from build123d import *

# Parameters (mm, degrees)
FILLET1_R = 0.635


with BuildPart() as part:
    # Sketch1 → Body (revolve)
    with BuildSketch(Plane.XY, mode=Mode.PRIVATE) as body_sk:
        with BuildLine():
            Line((-0.2794, 5.0038), (0, 5.0038))
            Line((0, 5.0038), (0, 2.38125))
            Line((0, 2.38125), (9.526, 2.38125))
            Line((9.526, 2.38125), (9.526, 3.602736))
            ThreePointArc((9.526, 3.602736), (11.862096638, 3.446669338), (14.098, 2.75209))
            Line((14.098, 2.75209), (14.098, 0))
            Line((14.098, 0), (-1.524, 0))
            ThreePointArc((-1.524, 0), (-1.208180863, 2.578131281), (-0.2794, 5.0038))
        make_face()
    revolve(body_sk.sketch.rotate(Axis((-1.524, 0, 0), (1, 0, 0)), 180), axis=Axis((-1.524, 0, 0), (1, 0, 0)))

    # Fillet1
    fillet1_edges = [part.edges().sort_by_distance(p)[0] for p in [
        (0, 2.38125, 0),
    ]]
    fillet(fillet1_edges, radius=FILLET1_R)


solid = part.part
Read the model definition and answer for the solid it produces. Units are mm, in the model's axes. Give positions to 0.01 mm unless a question says otherwise; leave off trailing zeros. Write each loop counter-clockwise with the first axis right and the second up, starting at its lowest first coordinate (ties: lowest second). Pieces come first, ordered by that corner, then holes. Notation, with made-up numbers: (69, 60) - (86, 60) arc R27 ccw to (86, 80) - close; hole circle Ø2 at (-33, -7.75). An arc over 180 degrees is marked (long way). Answer in a Markdown table with one row per item. Add a question column.
Item 1: Section C-C, the plane x = 0.25 is taken. Write down the section's boundary in (y, z), and give its area (3 significant figures).
Item 2: Flat-ended cylindrical pins translate along their axes: P1, Ø5, axis at y = -0.5, z = -1, coming from the -X side; P2, Ø3, axis at y = -3, z = -2.5, coming from the -X side; P3, Ø4, axis at y = -2.5, z = -3, coming from the -X side. Find the tip coordinate at first contact, or state that the pin passes through.
Item 3: Determine the mould class of faces 1 (the face through (9.526, -0.9, 2.4)), 2 (the face through (14.098, 0, 0)), 3 (the face through (5.143, 0.516, 2.325)) for opening direction X: pulls with the +X half, pulls with the -X half, needs draft (parallel to the pull), parting line crosses it, or undercut.
Item 4: Section B-B, the plane y = 4 is taken. Write down the section's boundary in (x, z), and give its area (3 significant figures).
Item 5: Find the intervals of material crossed by L1, parallel to Z at x = 0.25, y = 0.75; L2, parallel to Z at x = 10.5, y = -1.25; L3, parallel to Y at x = 9.25, z = 2, in increasing order.
Item 6: Section A-A, the plane x = 7 is taken. Write down the section's boundary in (y, z), and give its area (3 significant figures).
Recorded:
| question | item | result |
|---|---|---|
| 1 | outline | circle Ø5.02 at (0, 0) |
| 1 | area | 19.8 mm2 |
| 2 | P1 | stops at x = -1.52 |
| 2 | P2 | stops at x = -1.25 |
| 2 | P3 | stops at x = -1.35 |
| 3 | face 1 | undercut |
| 3 | face 2 | pulls with the +X half |
| 3 | face 3 | undercut |
| 4 | outline | (-0.28, -3.01) - (0, -3.01) - (0, 3.01) - (-0.28, 3.01) arc R9.9 ccw to start |
| 4 | area | 3.56 mm2 |
| 5 | L1 | z = -2.4 to 2.4 |
| 5 | L2 | z = -3.38 to 3.38 |
| 5 | L3 | y = -1.29 to 1.29 |
| 6 | outline | circle Ø4.76 at (0, 0) |
| 6 | area | 17.8 mm2 |
